Source: CAD feature listing. Evaluate the final solid. Frame: model axes, mm. A direction names the side the tool comes from. Give positions to 0.01 mm unless a question says otherwise; leave off trailing zeros. Loops run counter-clockwise (first coordinate to the right, second up) from the corner with the lowest first, then second, coordinate; pieces in that order, holes last.
from build123d import *

# Parameters (mm, degrees)
F0_R     = 9.525
F1_DEPTH = 25.4
F3_DEPTH = 25.401
F4_W     = 9.525
F4_H     = 9.723438
F5_DEPTH = 11.0998


with BuildPart() as f1:
    # F0 (on Front) → F1 (new body)
    with BuildSketch(Plane.XZ):
        Circle(F0_R)
    extrude(amount=F1_DEPTH)

    # F2 (on Front) → F3 (cut, through all)
    with BuildSketch(Plane.XZ):
        with BuildLine():
            ThreePointArc((4.7625, 0), (3.367596, 3.367596), (0, 4.7625))
            ThreePointArc((0, 4.7625), (-3.367596, 3.367596), (-4.7625, 0))
            ThreePointArc((-4.7625, 0), (-3.367596, -3.367596), (0, -4.7625))
            ThreePointArc((0, -4.7625), (3.367596, -3.367596), (4.7625, 0))
        make_face()
    extrude(amount=F3_DEPTH, mode=Mode.SUBTRACT)

    # F4 (on Front) → F5 (cut)
    with BuildSketch(Plane.XZ):
        Rectangle(F4_W, F4_H)
    extrude(amount=F5_DEPTH, mode=Mode.SUBTRACT)


solid = f1.part
1) Cut plane C-C (x = -3.75). Return loops of the section in (y, z), and give its area (3 significant figures).
Checks:
outline: (-25.4, -8.76) - (0, -8.76) - (0, -4.86) - (-11.1, -4.86) - (-11.1, -2.94) - (-25.4, -2.94) - close; (-25.4, 2.94) - (-11.1, 2.94) - (-11.1, 4.86) - (0, 4.86) - (0, 8.76) - (-25.4, 8.76) - close
area: 253 mm2
2) Cut plane A-A (z = 2.5). Return loops of the section in (x, y), and give its area (3 significant figures).
Checks:
outline: (-9.19, -25.4) - (-4.05, -25.4) - (-4.05, -11.1) - (-4.76, -11.1) - (-4.76, 0) - (-9.19, 0) - close; (4.05, -25.4) - (9.19, -25.4) - (9.19, 0) - (4.76, 0) - (4.76, -11.1) - (4.05, -11.1) - close
area: 245 mm2
3) Pull-direction query (X, two-part tool) for faces 1 (the flat face through (4.762, -5, 0)), 2 (the flat face through (-4.4, -25.4, 2.3)), 3 (the cylindrical face through (-7.559, -12.522, -5.796)), 4 (the flat face through (0, -5, -4.862)); classes: released by +X, released by -X, zero draft, split by the parting line, or undercut.
Checks:
face 1: undercut
face 2: zero draft
face 3: split by the parting line
face 4: undercut
4) Reachability of faces 5 (the flat face through (0, 0, -6)), 6 (the flat face through (-4.762, -5, 0)) from +Z, -Z, +X, -X, +Y, -Y: full face, straight path, thin tool, end or side. Return the list, or none.
Checks:
face 5: +Z, -Z, +X, -X, +Y
face 6: +Y
5) Ray query, probe 1 along X at (y, z) = (-17.5, 2); probe 2 along Z at (x, y) = (2.25, -14); probe 3 along Y at (x, z) = (-4.5, 4.5). Return the intervals inside material, ascending.
Checks:
probe 1: x = -9.31 to -4.32, 4.32 to 9.31
probe 2: z = -9.26 to -4.2, 4.2 to 9.26
probe 3: y = -25.4 to -11.1
6) Contact query for flat-ended pins moving along their axis: P1, Ø3, axis at x = 2, y = -4, coming from the -Z side; P2, Ø8, axis at y = -12, z = -5, coming from the +X side; P3, Ø6, axis at x = -7, y = -20, coming from the -Z side. Output: stop coordinate, or through.
Checks:
P1: stops at z = -9.51
P2: stops at x = 9.47
P3: stops at z = -8.64
